Read the model definition and answer for the solid it produces. Units are mm, in the model's axes. Face numbers are marked on the shaded views. A direction names the side the tool comes from. Give positions to 0.01 mm unless a question says otherwise; leave off trailing zeros. Write each loop counter-clockwise with the first axis right and the second up, starting at its lowest first coordinate (ties: lowest second). Pieces come first, ordered by that corner, then holes.
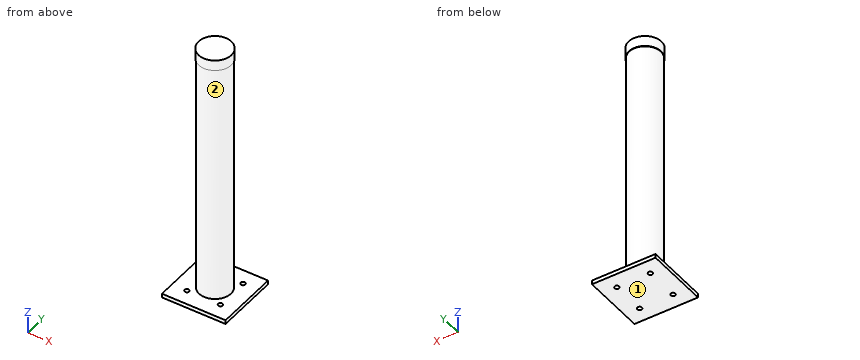
```python
from build123d import *

# Parameters (mm, degrees)
F0_R     = 38.1
F0_R_2   = 34.925
F1_DEPTH = 609.6
F2_W     = 152.4
F2_H     = 152.4
F2_R     = 5.489771
F3_DEPTH = 9.525
F4_R     = 39.285427
F5_DEPTH = 25.4


with BuildPart() as f1:
    # F0 (on Top) → F1 (new body)
    with BuildSketch(Plane.XY):
        Circle(F0_R)
        Circle(F0_R_2, mode=Mode.SUBTRACT)
    extrude(amount=F1_DEPTH)

    # F2 (on Top) → F3 (join)
    with BuildSketch(Plane.XY):
        Rectangle(F2_W, F2_H)
        with Locations((-40.11862, -40.534951)):
            Circle(F2_R, mode=Mode.SUBTRACT)
        with Locations((40.11862, -40.534951)):
            Circle(F2_R, mode=Mode.SUBTRACT)
        with Locations((-40.11862, 40.534951)):
            Circle(F2_R, mode=Mode.SUBTRACT)
        with Locations((40.11862, 40.534951)):
            Circle(F2_R, mode=Mode.SUBTRACT)
    extrude(amount=-F3_DEPTH)

    # F4 (on face) → F5 (join)
    with BuildSketch(Plane.XY.offset(609.6)):
        Circle(F4_R)
    extrude(amount=-F5_DEPTH)


solid = f1.part
```
Item 1: Section C-C (z = 73) is taken. Write down the section's boundary in (x, y) (3 decimals), and give its area (3 significant figures).
Result set:
outline: circle Ø76.2 at (0, 0); hole circle Ø69.85 at (0, 0)
area: 728 mm2
Item 2: Which of the six approach directions +Z, -Z, +X, -X, +Y, -Y give full straight-line access (tool end or side, diameter ignored) to the marked faces 1 and 2?
Result set:
face 1: -Z, +X, -X, +Y, -Y
face 2: none
Item 3: Section D-D (y = 57) is taken. Write down the section's boundary in (x, z) (3 decimals), and give its area (3 significant figures).
Result set:
outline: (-76.2, -9.525) - (76.2, -9.525) - (76.2, 0) - (-76.2, 0) - close
area: 1,450 mm2
Item 4: Each of these flat-tipped pins is pushed along its axis until it touches: pin 1 Ø8 at (y, z) = (2.5, 273) entering from -X; pin 2 Ø5 at (x, z) = (29.5, 406.5) entering from -Y; pin 3 Ø1.5 at (x, z) = (-22.5, 424.5) entering from +Y. Where does it stop, or does it pass through?
Result set:
pin 1: stops at x = -38.1
pin 2: stops at y = -26.88
pin 3: stops at y = 31.28
Item 5: Section A-A (x = 0) is taken. Write down the section's boundary in (y, z) (3 decimals).
Result set:
outline: (-76.2, -9.525) - (76.2, -9.525) - (76.2, 0) - (38.1, 0) - (38.1, 584.2) - (39.285, 584.2) - (39.285, 609.6) - (-39.285, 609.6) - (-39.285, 584.2) - (-38.1, 584.2) - (-38.1, 0) - (-76.2, 0) - close; hole (-34.925, 0) - (34.925, 0) - (34.925, 584.2) - (-34.925, 584.2) - close
Item 6: Find the intervals of material crossed by line 1 along X through (y, z) = (-3, 465); line 2 along Y through (x, z) = (0, 405.5) (3 decimals); line 3 along Z through (x, y) = (21, -5.5) (3 decimals), in increasing order.
Result set:
line 1: x = -37.98 to -34.8, 34.8 to 37.98
line 2: y = -38.1 to -34.925, 34.925 to 38.1
line 3: z = -9.525 to 0, 584.2 to 609.6
